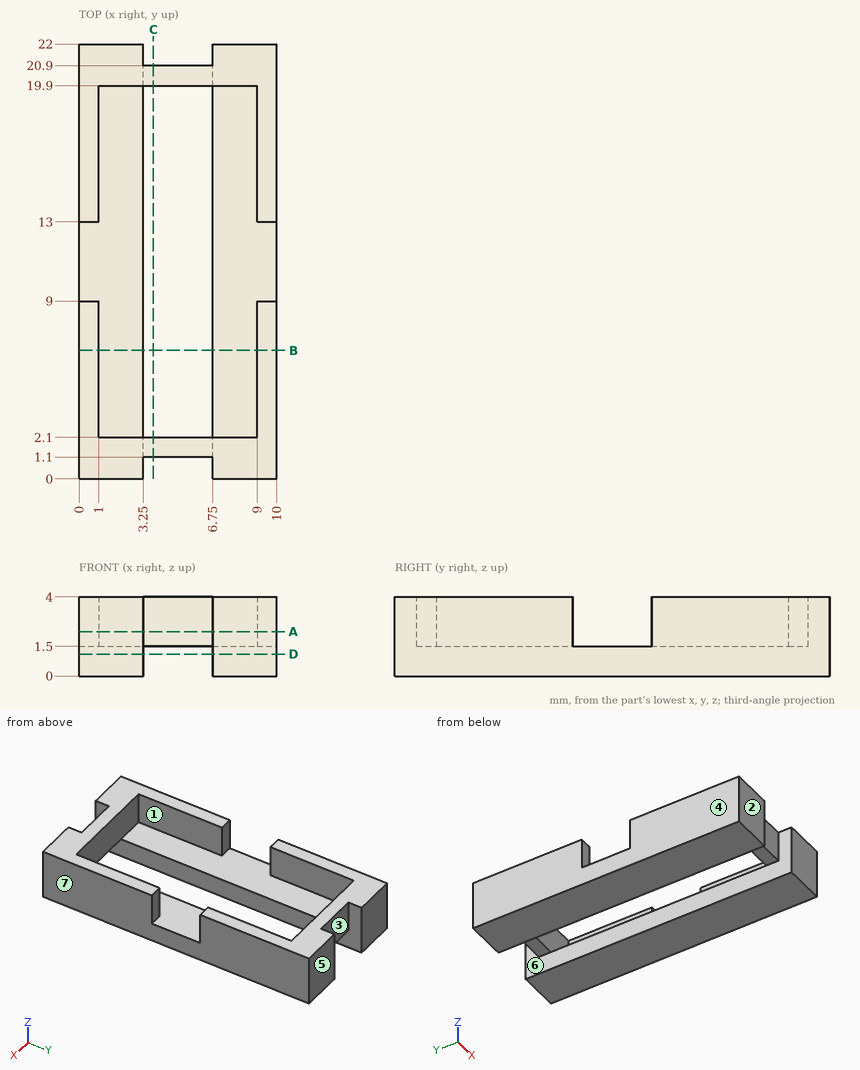
Source: three-view drawing plus pictorial views. Frame: mm from the lowest corner of the part. A direction names the side the tool comes from. Round coordinates to 2 decimals unless told otherwise and drop trailing zeros. Write each loop counter-clockwise with the first axis right and the second up, starting at its lowest first coordinate (ties: lowest second). Pieces come first, ordered by that corner, then holes. Notation, with made-up numbers: M 82.25,68.25 L 93.25,68.25 A22 ccw 93.25,91.25 Z; hole C -19.75,-34 d10. An arc over 180 degrees is marked long. Use CSV: the item, a comma, the result in double quotes. Start each with the question number.
Q1. First-contact query: P1, Ø1.1, axis at x = 4.5, y = 1.5, coming from the -Z side; P2, Ø3.5, axis at x = 1.5, y = 13, coming from the +Z side; P3, Ø1, axis at x = 4.5, y = 18, coming from the -Z side. Flat tips, straight axial feed; report the tip coordinate or a pass-through.
Q2. Pull-direction query (X, two-part tool) for the marked faces 4, 5, 6 and 7; classes: +X half, -X half, draft (parallel to the pull), parting line (faces both ways), or undercut.
Q3. Cut plane B-B on y = 6.5. Output: boundary loops of the cut face in (x, z), plus the area to 4 significant figures.
Q4. Cut plane A-A on z = 2.25. Output: boundary loops of the cut face in (x, y), plus the area to 3 significant figures.
Q5. Access query for the marked faces 1, 2 and 3. Directions: +Z, -Z, +X, -X, +Y, -Y. A direction counts if a zero-diameter tool reaches every point of the face in a straight line with its end or side. Return the directions, or none.
Q6. Cut plane D-D on z = 1.1. Output: boundary loops of the cut face in (x, y), plus the area to 3 significant figures.
Q7. Cut plane C-C on x = 3.75. Output: boundary loops of the cut face in (y, z).
Q8. Line query: line 1 (X direction, y = 13.25, z = 1.6); line 2 (Y direction, x = 8.5, z = 3.7); line 3 (X direction, y = 4.5, z = 1.15). Output: solid intervals per line, ascending. Write a range as from..to.
Results found:
1,P1,"z = 1.5"
1,P2,"z = 4"
1,P3,"through"
2,face 4,"-X half"
2,face 5,"draft"
2,face 6,"undercut"
2,face 7,"+X half"
3,outline,"M 0,0 L 3.25,0 L 3.25,1.5 L 1,1.5 L 1,4 L 0,4 Z; M 6.75,0 L 10,0 L 10,4 L 9,4 L 9,1.5 L 6.75,1.5 Z"
3,area,"14.75 mm^2"
4,outline,"M 0,0 L 3.25,0 L 3.25,1.1 L 6.75,1.1 L 6.75,0 L 10,0 L 10,9 L 9,9 L 9,2.1 L 1,2.1 L 1,9 L 0,9 Z; M 0,13 L 1,13 L 1,19.9 L 9,19.9 L 9,13 L 10,13 L 10,22 L 6.75,22 L 6.75,20.9 L 3.25,20.9 L 3.25,22 L 0,22 Z"
4,area,"61.9 mm^2"
5,face 1,"+Z"
5,face 2,"+Z, -Z, +X, -X, -Y"
5,face 3,"+Z, -Z, +Y"
6,outline,"M 0,0 L 3.25,0 L 3.25,22 L 0,22 Z; M 6.75,0 L 10,0 L 10,22 L 6.75,22 Z"
6,area,"143 mm^2"
7,outline,"M 1.1,1.5 L 2.1,1.5 L 2.1,4 L 1.1,4 Z; M 19.9,1.5 L 20.9,1.5 L 20.9,4 L 19.9,4 Z"
8,line 1,"0..1, 9..10"
8,line 2,"0..2.1, 19.9..22"
8,line 3,"0..3.25, 6.75..10"
